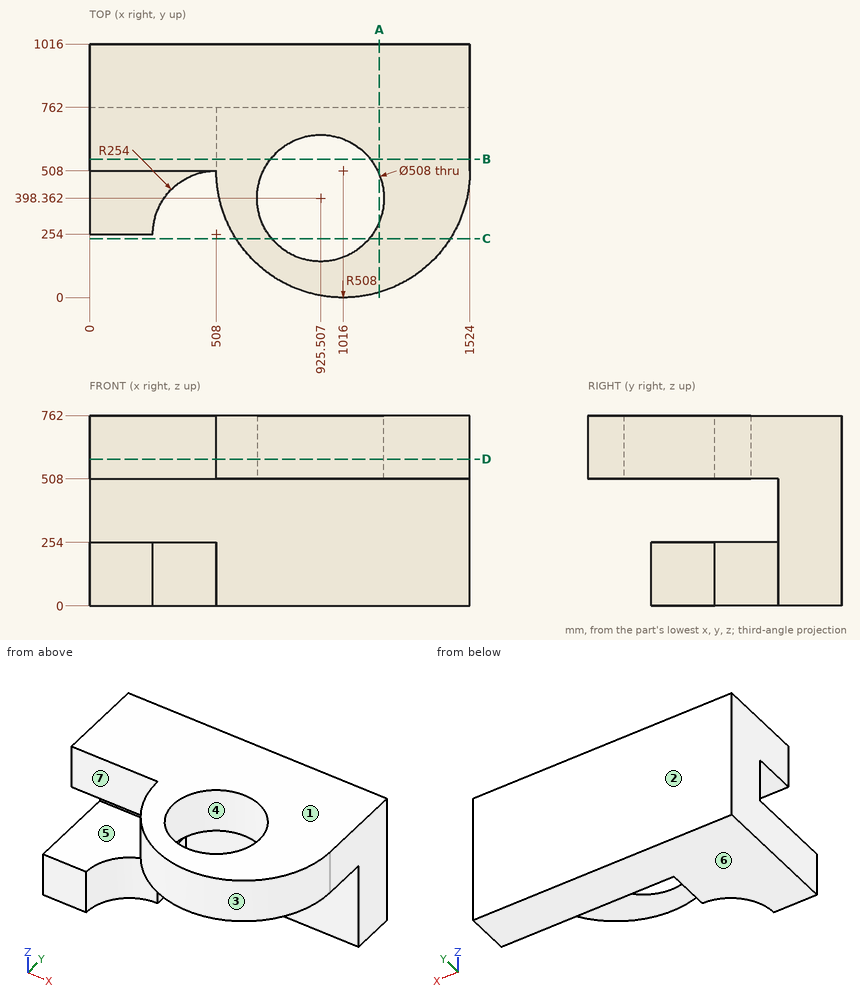
Geometry check sheet. Reference: drawing and pictorial views, mm from the part's lowest x, y, z. A direction names the side the tool comes from. Round coordinates to 2 decimals unless told otherwise and drop trailing zeros. Order: outer loops, then holes, each group sorted by start corner. A loop starts at its lowest first (then second) coordinate and runs counter-clockwise, first axis right, second up. Notation, with made-up numbers: (19.25, 30) -> (51.25, 30) arc R21 cw to (51.25, 36) -> close; hole circle Ø9 at (-32.75, 19). An arc over 180 degrees is marked (long way). One line per item, written item: value. Start each with the question number.
Q1. Gauge pin test, flat ends, axial feed: pin 1 Ø6 at (x, z) = (793, 466.5) entering from -Y; pin 2 Ø4 at (x, y) = (669, 444.5) entering from -Z; pin 3 Ø8 at (y, z) = (263.5, 562.5) entering from +X. Record the tip position at first contact, or that the pin passes through.
Q2. Cross-section at C-C (y = 236). Record the boundary of the cut face in (x, z) (1 decimal).
Q3. Cross-section at D-D (z = 587.5). Record the boundary of the cut face in (x, y), and give its area (3 significant figures).
Q4. Thickness scan on line 1 (Z direction, x = 69, y = 646.5); line 2 (Y direction, x = 225, z = 688.5); line 3 (Y direction, x = 213, z = 491). Record the ranges inside material, lowest first.
Q5. Set-up check for the marked faces 5, 6 and 7: record each of +Z, -Z, +X, -X, +Y, -Y from which the full face is reachable in a straight line by a thin tool's end or side.
Q6. Cross-section at A-A (x = 1161.5). Record the boundary of the cut face in (y, z) (1 decimal).
Q7. Mould release check, pull along Y, two halves, no side actions. Record for the marked faces 1, 2, 3 and 4: pulls with the +Y half, pulls with the -Y half, needs draft (parallel to the pull), parting line crosses it, or undercut.
Q8. Cross-section at B-B (y = 555). Record the boundary of the cut face in (x, z), and give its area (3 significant figures).
Completed:
1. pin 1: stops at y = 762
1. pin 2: stops at z = 508
1. pin 3: stops at x = 1463.46
2. outline: (587, 508) -> (730.2, 508) -> (730.2, 762) -> (587, 762) -> close; (1120.8, 508) -> (1445, 508) -> (1445, 762) -> (1120.8, 762) -> close
3. outline: (0, 508) -> (508, 508) arc R508 ccw to (1524, 508) -> (1524, 1016) -> (0, 1016) -> close; hole circle Ø508 at (925.51, 398.36)
3. area: 977,000 mm²
4. line 1: z = 0 to 254, 508 to 762
4. line 2: y = 508 to 1016
4. line 3: y = 762 to 1016
5. face 5: +X, -X, -Y
5. face 6: -Z, +X, -X, +Y, -Y
5. face 7: +Z, -X, -Y
6. outline: (21.3, 508) -> (304.4, 508) -> (304.4, 762) -> (21.3, 762) -> close; (492.3, 508) -> (762, 508) -> (762, 0) -> (1016, 0) -> (1016, 762) -> (492.3, 762) -> close
7. face 1: needs draft
7. face 2: pulls with the +Y half
7. face 3: pulls with the -Y half
7. face 4: undercut
8. outline: (0, 0) -> (508, 0) -> (508, 254) -> (0, 254) -> close; (0, 508) -> (725.56, 508) -> (725.56, 762) -> (0, 762) -> close; (1125.46, 508) -> (1524, 508) -> (1524, 762) -> (1125.46, 762) -> close
8. area: 415,000 mm²
